Geometry: final body of the model. Coordinates: model frame, mm. A direction names the side the tool comes from. Coordinates: 2 decimals unless noted, no trailing zeros. Loops run counter-clockwise (first coordinate to the right, second up) from the corner with the lowest first, then second, coordinate; pieces in that order, holes last. Notation, with made-up numbers: (-2, 44.25) - (38, 44.25) arc R15 cw to (38, 70.25) - close; hole circle Ø3 at (14.25, 2). An arc over 180 degrees is marked (long way). Put each result on its own line as item: value. Start each with the question number.
1) Contact query for flat-ended pins moving along their axis: pin 1 Ø3 at (x, z) = (-17.5, -12) entering from -Y; pin 2 Ø1.8 at (x, z) = (8, 0) entering from -Y; pin 3 Ø1 at (y, z) = (-1, 6.5) entering from +X. Output: stop coordinate, or through.
2) Draft query along X for faces 1 (the flat face through (0.4, -3.3, 5.4)), 2 (the cylindrical face through (-15.821, 0.644, -20.633)), 3 (the cylindrical face through (18.329, -1.673, 7.253)). Return one class per face: +X half, -X half, draft (parallel to the pull), parting line (faces both ways), or undercut.
3) Material intervals for line 1 along X through (y, z) = (2.25, -10.5); line 2 along Z through (x, y) = (-21, -2.75); line 3 along X through (y, z) = (-1.4, 10.5), sorted ascending. Write a range as from..to.
4) Section B-B on z = 0. Output: boundary loops of the cut face in (x, y), and give its area (3 significant figures).
5) Section A-A on x = 0. Count the separate pieces of the cut face and the enclosed holes in it, and give its area (3 significant figures).
6) Reachability of faces 4 (the cylindrical face through (16.678, 2.317, 11.284)), 5 (the flat face through (-1.4, 0, 22.4)) from +Z, -Z, +X, -X, +Y, -Y: full face, straight path, thin tool, end or side. Return the list, or none.
7) Section C-C on z = -21. Output: boundary loops of the cut face in (x, y).
```python
from build123d import *

# Parameters (mm, degrees)
SKETCH1_R           = 26
SKETCH1_R_2         = 5
SKETCH1_R_3         = 1.7
SKETCH1_R_4         = 1.5
BOSS_EXTRUDE1_DEPTH = 4.7
BOSS_EXTRUDE2_START = -3.3
SKETCH1_3_R         = 26
SKETCH1_3_R_2       = 3.25
SKETCH1_3_R_3       = 1.5
SKETCH1_3_R_4       = 5
BOSS_EXTRUDE2_DEPTH = 3.3


with BuildPart() as part:
    # Sketch1 → Boss-Extrude1 (new body)
    with BuildSketch(Plane(origin=(0, 0, 0), x_dir=(1, 0, 0), z_dir=(0, 1, 0))):
        with Locations(Location((0, 0, 0), (0, 0, 270))):
            Circle(SKETCH1_R)
        with Locations(Location((0, 0, 0), (0, 0, 270))):
            Circle(SKETCH1_R_2, mode=Mode.SUBTRACT)
        with Locations(Location((0, 21, 0), (0, 0, 270))):
            Circle(SKETCH1_R_3, mode=Mode.SUBTRACT)
        with Locations(Location((18.186533479, 10.5, 0), (0, 0, 270))):
            Circle(SKETCH1_R_3, mode=Mode.SUBTRACT)
        with Locations(Location((18.186533479, -10.5, 0), (0, 0, 270))):
            Circle(SKETCH1_R_3, mode=Mode.SUBTRACT)
        with Locations(Location((0, -21, 0), (0, 0, 270))):
            Circle(SKETCH1_R_3, mode=Mode.SUBTRACT)
        with Locations(Location((-18.186533479, -10.5, 0), (0, 0, 270))):
            Circle(SKETCH1_R_3, mode=Mode.SUBTRACT)
        with Locations(Location((-18.186533479, 10.5, 0), (0, 0, 270))):
            Circle(SKETCH1_R_3, mode=Mode.SUBTRACT)
        with Locations(Location((0, -8, 0), (0, 0, 270))):
            Circle(SKETCH1_R_4, mode=Mode.SUBTRACT)
        with Locations(Location((-8, 0, 0), (0, 0, 270))):
            Circle(SKETCH1_R_4, mode=Mode.SUBTRACT)
        with Locations(Location((0, 8, 0), (0, 0, 270))):
            Circle(SKETCH1_R_4, mode=Mode.SUBTRACT)
        with Locations(Location((8, 0, 0), (0, 0, 270))):
            Circle(SKETCH1_R_4, mode=Mode.SUBTRACT)
    extrude(amount=BOSS_EXTRUDE1_DEPTH)

    # Sketch1_3 → Boss-Extrude2 (add)
    with BuildSketch(Plane(origin=(0, 0, 0), x_dir=(1, 0, 0), z_dir=(0, 1, 0)).offset(BOSS_EXTRUDE2_START)):
        with Locations(Location((0, 0, 0), (0, 0, 270))):
            Circle(SKETCH1_3_R)
        with Locations(Location((-18.186533479, 10.5, 0), (0, 0, 270))):
            Circle(SKETCH1_3_R_2, mode=Mode.SUBTRACT)
        with Locations(Location((-18.186533479, -10.5, 0), (0, 0, 270))):
            Circle(SKETCH1_3_R_2, mode=Mode.SUBTRACT)
        with Locations(Location((0, -21, 0), (0, 0, 270))):
            Circle(SKETCH1_3_R_2, mode=Mode.SUBTRACT)
        with Locations(Location((18.186533479, -10.5, 0), (0, 0, 270))):
            Circle(SKETCH1_3_R_2, mode=Mode.SUBTRACT)
        with Locations(Location((18.186533479, 10.5, 0), (0, 0, 270))):
            Circle(SKETCH1_3_R_2, mode=Mode.SUBTRACT)
        with Locations(Location((0, 21, 0), (0, 0, 270))):
            Circle(SKETCH1_3_R_2, mode=Mode.SUBTRACT)
        with Locations(Location((8, 0, 0), (0, 0, 270))):
            Circle(SKETCH1_3_R_3, mode=Mode.SUBTRACT)
        with Locations(Location((0, 8, 0), (0, 0, 270))):
            Circle(SKETCH1_3_R_3, mode=Mode.SUBTRACT)
        with Locations(Location((-8, 0, 0), (0, 0, 270))):
            Circle(SKETCH1_3_R_3, mode=Mode.SUBTRACT)
        with Locations(Location((0, -8, 0), (0, 0, 270))):
            Circle(SKETCH1_3_R_3, mode=Mode.SUBTRACT)
        with Locations(Location((0, 0, 0), (0, 0, 270))):
            Circle(SKETCH1_3_R_4, mode=Mode.SUBTRACT)
    extrude(amount=BOSS_EXTRUDE2_DEPTH)


solid = part.part
```
Answer block:
1. pin 1: stops at y = 0
1. pin 2: passes through
1. pin 3: stops at x = 25.3
2. face 1: draft
2. face 2: parting line
2. face 3: undercut
3. line 1: x = -23.79..-19.89, -16.49..16.49, 19.89..23.79
3. line 2: z = -15.33..-12.13, -8.87..8.87, 12.13..15.33
3. line 3: x = -23.79..-21.44, -14.94..14.94, 21.44..23.79
4. outline: (-26, -3.3) - (-9.5, -3.3) - (-9.5, 4.7) - (-26, 4.7) - close; (-6.5, -3.3) - (-5, -3.3) - (-5, 4.7) - (-6.5, 4.7) - close; (5, -3.3) - (6.5, -3.3) - (6.5, 4.7) - (5, 4.7) - close; (9.5, -3.3) - (26, -3.3) - (26, 4.7) - (9.5, 4.7) - close
4. area: 288 mm²
5. separate pieces: 6
5. enclosed holes: 0
5. area: 213 mm²
6. face 4: +Y, -Y
6. face 5: -Y
7. outline: (-15.33, -3.3) - (-3.25, -3.3) - (-3.25, 0) - (-1.7, 0) - (-1.7, 4.7) - (-15.33, 4.7) - close; (1.7, 0) - (3.25, 0) - (3.25, -3.3) - (15.33, -3.3) - (15.33, 4.7) - (1.7, 4.7) - close
